from build123d import *

# Parameters (mm, degrees)
EXTRUDE_1_DEPTH             = 90
SKETCH_2_W                  = 90
SKETCH_2_H                  = 17.75
EXTRUDE_2_DEPTH             = 8.2
SKETCH_3_W                  = 90
SKETCH_3_H                  = 50.95
EXTRUDE_3_DEPTH             = 8.2
SKETCH_4_W                  = 3.95
SKETCH_4_H                  = 29.5
CUT_EXTRUDE_1_DEPTH         = 96.44153315
SKETCH_5_W                  = 3.95
SKETCH_5_H                  = 6.2
CUT_EXTRUDE_2_DEPTH         = 96.44153315
SKETCH_6_W                  = 2.25
SKETCH_6_H                  = 3.95
CUT_EXTRUDE_3_DEPTH         = 96.44153315
SKETCH_7_W                  = 4.5
SKETCH_7_H                  = 3.95
CUT_EXTRUDE_4_DEPTH         = 96.44153315
SKETCH_8_W                  = 2.25
SKETCH_8_H                  = 3.95
CUT_EXTRUDE_5_DEPTH         = 96.44153315
SKETCH_9_W                  = 3.95
SKETCH_9_H                  = 2.25
CUT_EXTRUDE_6_DEPTH         = 96.44153315
SKETCH_10_W                 = 20.2
SKETCH_10_H                 = 45.2
CUT_EXTRUDE_7_DEPTH         = 86
HOLE_WIZARD_2_5_2_5_1_D     = 2.5
HOLE_WIZARD_4_5_4_5_1_D     = 4.5
HOLE_WIZARD_8_3_8_3_1_D     = 8.3
HOLE_WIZARD_8_3_8_3_1_DEPTH = 3.2
FILLET_1_R                  = 2
FILLET_2_R                  = 2
EXTRUDE_START               = -90
SKETCH_17_R                 = 1.25
EXTRUDE_4_DEPTH             = 90
CUT_EXTRUDE_START           = -100
SKETCH_18_R                 = 4.15
CUT_EXTRUDE_8_DEPTH         = 100
CUT_EXTRUDE_9_DEPTH         = 110
CUT_EXTRUDE_10_DEPTH        = 110
SKETCH_21_W                 = 90
SKETCH_21_H                 = 47
EXTRUDE_5_DEPTH             = 2


with BuildPart() as part:
    # Эскиз1 → Бобышка-Вытянуть1 (new body)
    with BuildSketch(Plane(origin=(90, 0, 0), x_dir=(0, 0, -1), z_dir=(1, 0, 0))):
        with BuildLine():
            Line((6.75, -24.093761792), (6.75, 19.25))
            Line((6.75, 19.25), (-11.593761792, 19.25))
            ThreePointArc((-11.593761792, 19.25), (-15.325, 18), (-11.593761792, 16.75))
            Line((-11.593761792, 16.75), (-11, 16.75))
            Line((-11, 16.75), (-11, -16.75))
            Line((-11, -16.75), (-11.593761792, -16.75))
            ThreePointArc((-11.593761792, -16.75), (-15.325, -18), (-11.593761792, -19.25))
            Line((-11.593761792, -19.25), (-11, -19.25))
            Line((-11, -19.25), (-11, -23.5))
            Line((-11, -23.5), (-6.75, -23.5))
            Line((-6.75, -23.5), (-6.75, -24.093761792))
            ThreePointArc((-6.75, -24.093761792), (-5.5, -27.825), (-4.25, -24.093761792))
            Line((-4.25, -24.093761792), (-4.25, -23.5))
            Line((-4.25, -23.5), (4.25, -23.5))
            Line((4.25, -23.5), (4.25, -24.093761792))
            ThreePointArc((4.25, -24.093761792), (5.5, -27.825), (6.75, -24.093761792))
        make_face()
    extrude(amount=-EXTRUDE_1_DEPTH)

    # Эскиз2 → Бобышка-Вытянуть2 (add)
    with BuildSketch(Plane(origin=(0, 19.25, 0), x_dir=(-1, 0, 0), z_dir=(0, 1, 0))):
        with Locations((-45, 2.125)):
            Rectangle(SKETCH_2_W, SKETCH_2_H)
    extrude(amount=EXTRUDE_2_DEPTH)

    # Эскиз3 → Бобышка-Вытянуть3 (add)
    with BuildSketch(Plane(origin=(0, 0, -6.75), x_dir=(-1, 0, 0), z_dir=(0, 0, -1))):
        with Locations((-45, 1.975)):
            Rectangle(SKETCH_3_W, SKETCH_3_H)
    extrude(amount=EXTRUDE_3_DEPTH)

    # Эскиз4 → Вырез-Вытянуть1 (cut, through all)
    with BuildSketch(Plane.ZY):
        with Locations((-12.975, 0)):
            Rectangle(SKETCH_4_W, SKETCH_4_H)
    extrude(amount=-CUT_EXTRUDE_1_DEPTH, mode=Mode.SUBTRACT)

    # Эскиз5 → Вырез-Вытянуть2 (cut, through all)
    with BuildSketch(Plane.ZY):
        with Locations((-12.975, 24.35)):
            Rectangle(SKETCH_5_W, SKETCH_5_H)
    extrude(amount=-CUT_EXTRUDE_2_DEPTH, mode=Mode.SUBTRACT)

    # Эскиз6 → Вырез-Вытянуть3 (cut, through all)
    with BuildSketch(Plane.ZY):
        with Locations((-9.875, 25.475)):
            Rectangle(SKETCH_6_W, SKETCH_6_H)
    extrude(amount=-CUT_EXTRUDE_3_DEPTH, mode=Mode.SUBTRACT)

    # Эскиз7 → Вырез-Вытянуть4 (cut, through all)
    with BuildSketch(Plane.ZY):
        with Locations((0, 25.475)):
            Rectangle(SKETCH_7_W, SKETCH_7_H)
    extrude(amount=-CUT_EXTRUDE_4_DEPTH, mode=Mode.SUBTRACT)

    # Эскиз8 → Вырез-Вытянуть5 (cut, through all)
    with BuildSketch(Plane.ZY):
        with Locations((9.875, 25.475)):
            Rectangle(SKETCH_8_W, SKETCH_8_H)
    extrude(amount=-CUT_EXTRUDE_5_DEPTH, mode=Mode.SUBTRACT)

    # Эскиз9 → Вырез-Вытянуть6 (cut, through all)
    with BuildSketch(Plane.ZY):
        with Locations((-12.975, -22.375)):
            Rectangle(SKETCH_9_W, SKETCH_9_H)
    extrude(amount=-CUT_EXTRUDE_6_DEPTH, mode=Mode.SUBTRACT)

    # Эскиз10 → Вырез-Вытянуть7 (cut)
    with BuildSketch(Plane(origin=(90, 0, 0), x_dir=(0, 0, -1), z_dir=(1, 0, 0))):
        Rectangle(SKETCH_10_W, SKETCH_10_H)
    extrude(amount=-CUT_EXTRUDE_7_DEPTH, mode=Mode.SUBTRACT)

    # Диаметр отверстия Ø2.5 (2.5)1 (through all)
    with Locations(Plane(origin=(90, 0, 0), x_dir=(0, 0, -1), z_dir=(1, 0, 0))):
        with Locations((5.5, -25.75), (-13.25, -18), (-5.5, -25.75), (-13.25, 18)):
            Hole(HOLE_WIZARD_2_5_2_5_1_D / 2)

    # Диаметр отверстия Ø4.5 (4.5)1 (through all)
    with Locations(Plane.ZY):
        with Locations((-13.25, -18), (-13.25, 18), (-5.5, 25.75), (5.5, 25.75)):
            Hole(HOLE_WIZARD_4_5_4_5_1_D / 2)

    # Диаметр отверстия Ø8.3 (8.3)1
    with Locations(Plane.ZY):
        with Locations((0, 0)):
            Hole(HOLE_WIZARD_8_3_8_3_1_D / 2, depth=HOLE_WIZARD_8_3_8_3_1_DEPTH)

    # Скругление1
    fillet_1_edges = [part.edges().sort_by_distance(p)[0] for p in [
        (45, 23.5, 8.75),
    ]]
    fillet(fillet_1_edges, radius=FILLET_1_R)

    # Скругление2
    fillet_2_edges = [part.edges().sort_by_distance(p)[0] for p in [
        (45, 23.5, -8.75),
        (45, 23.5, 2.25),
        (45, 23.5, -2.25),
        (45, -21.25, -11),
        (4, 0, -10.1),
        (4, -22.6, 0),
        (4, 0, 10.1),
        (4, 22.6, 0),
        (45, 14.75, -11),
        (45, -14.75, -11),
        (45, 21.25, -11),
    ]]
    fillet(fillet_2_edges, radius=FILLET_2_R)

    # Эскиз17 → Бобышка-Вытянуть4 (add)
    with BuildSketch(Plane(origin=(90, 0, 0), x_dir=(0, 0, -1), z_dir=(1, 0, 0)).offset(EXTRUDE_START)):
        with Locations((5.5, -25.75)):
            Circle(SKETCH_17_R)
        with Locations((-5.5, -25.75)):
            Circle(SKETCH_17_R)
        with Locations((-13.25, -18)):
            Circle(SKETCH_17_R)
        with Locations((-13.25, 18)):
            Circle(SKETCH_17_R)
    extrude(amount=EXTRUDE_4_DEPTH)

    # Эскиз18 → Вырез-Вытянуть8 (cut)
    with BuildSketch(Plane.ZY.offset(CUT_EXTRUDE_START)):
        Circle(SKETCH_18_R)
    extrude(amount=CUT_EXTRUDE_8_DEPTH, mode=Mode.SUBTRACT)

    # Эскиз19 → Вырез-Вытянуть9 (cut)
    with BuildSketch(Plane(origin=(90, 0, 0), x_dir=(0, 0, -1), z_dir=(1, 0, 0))):
        Polygon((10.1, -22.6), (10.1, 22.6), (10.1, 31.019338608), (-21.722605493, 31.019338608), (-21.722605493, -29.745467662), (10.1, -29.745467662), align=None)
    extrude(amount=-CUT_EXTRUDE_9_DEPTH, mode=Mode.SUBTRACT)

    # Эскиз20 → Вырез-Вытянуть10 (cut)
    with BuildSketch(Plane(origin=(90, 0, 0), x_dir=(0, 0, -1), z_dir=(1, 0, 0))):
        with BuildLine():
            Line((10.1, 23.5), (10.1, 23.608571968))
            ThreePointArc((10.1, 23.608571968), (10.420497393, 23.52732972), (10.75, 23.5))
            Line((10.75, 23.5), (10.1, 23.5))
        make_face()
    extrude(amount=-CUT_EXTRUDE_10_DEPTH, mode=Mode.SUBTRACT)

    # Эскиз21 → Бобышка-Вытянуть5 (add)
    with BuildSketch(Plane.XY.offset(-10.1)):
        with Locations((45, 0)):
            Rectangle(SKETCH_21_W, SKETCH_21_H)
    extrude(amount=EXTRUDE_5_DEPTH)


solid = part.part
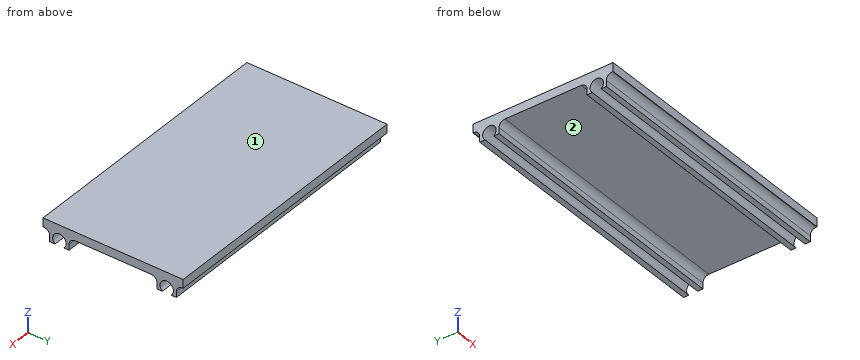
Could you check a few things on this model? Use its own coordinates, in mm. Face numbers are marked on the shaded views. A direction names the side the tool comes from. Coordinates: 2 decimals unless noted, no trailing zeros. Order: outer loops, then holes, each group sorted by start corner. A loop starts at its lowest first (then second) coordinate and runs counter-clockwise, first axis right, second up.
Q1. Suppose I cut it at A-A on x = 27.5. Please give me the cut outline in (y, z).
Q2. Suppose I cut it at B-B on y = 8.5. Please give me the cut outline in (x, z).
Q3. Will these pins go through, and if not, where does the flat tip stop? pin 1 (1 mm diameter, centred on x = 32.5, z = -14.5, fed in from -Y); pin 2 (4 mm diameter, centred on x = 23.5, z = -13.5, fed in from -Y); pin 3 (1 mm diameter, centred on x = 48, z = -12.5, fed in from +Y).
Q4. Please list where these lines run through material, in increasing order: L1, parallel to Y at x = 52, z = -13.25; L2, parallel to Y at x = 83.5, z = -13; L3, parallel to Z at x = 8, y = 8.
Q5. Which directions (+Z, -Z, +X, -X, +Y, -Y) give clear straight access to the entire face, cutting with the end or side of a thin tool? Please do the marked faces 1 and 2.
Answer:
1. outline: (-23.5, -11) - (-23.25, -11) arc R2 cw to (-21.25, -13) - (-21.25, -14.95) - (-19.47, -14.95) arc R2.25 cw (long way) to (-16.53, -14.95) - (-14.75, -14.95) - (-14.75, -13) arc R2 cw to (-12.75, -11) - (12.75, -11) arc R2 cw to (14.75, -13) - (14.75, -14.95) - (16.53, -14.95) arc R2.25 cw (long way) to (19.47, -14.95) - (21.25, -14.95) - (21.25, -13) arc R2 cw to (23.25, -11) - (23.5, -11) - (23.5, -8.1) - (-23.5, -8.1) - close
2. outline: (0, -11) - (90, -11) - (90, -8.1) - (0, -8.1) - close
3. pin 1: stops at y = -21.25
3. pin 2: stops at y = -21.93
3. pin 3: stops at y = 21.52
4. L1: y = -21.25 to -20.25, -15.75 to -14.75, 14.75 to 15.75, 20.25 to 21.25
4. L2: y = -21.25 to -20.24, -15.76 to -14.75, 14.75 to 15.76, 20.24 to 21.25
4. L3: z = -11 to -8.1
5. face 1: +Z, +X, -X, +Y, -Y
5. face 2: -Z, +X, -X
